```python
from build123d import *

# Parameters (mm, degrees)
F0_R            = 6.035
F1_DEPTH        = 3.175
F3_COPIES_COUNT = 2
F4_T3_ANGLE     = 67.6677552602
F4_T6_ANGLE     = 67.6677552602
F4_T9_ANGLE     = 135.3490310549
F4_T18_ANGLE    = 135.3490310549
F4_T21_ANGLE    = 67.6677552602
F4_T24_ANGLE    = 67.6677552602
F5_R            = 1.27


# Not quite as in the source:
# - a fillet or chamfer that OpenCascade refuses, or shapes differently, is made with other operations: its cross-section is extruded or revolved along the edge and cut away or added
# - a pattern or mirror of a feature is missing from the dataset's text; its kind, count and spacing are read off the source's solid


with BuildPart() as f1:
    # F0 (on Top) → F1 (new body, symmetric)
    with BuildSketch(Plane.XY):
        with BuildLine():
            Line((18.2389864028, 12.7), (-18.2389864028, 12.7))
            ThreePointArc((-18.2389864028, 12.7), (-22.225, 0), (-18.2389864028, -12.7))
            Line((-18.2389864028, -12.7), (18.2389864028, -12.7))
            ThreePointArc((18.2389864028, -12.7), (22.225, 0), (18.2389864028, 12.7))
        make_face()
        Circle(F0_R, mode=Mode.SUBTRACT)
    extrude(amount=F1_DEPTH, both=True)

    # F2 (on Front) → F3 (revolve, cut)
    with BuildSketch(Plane.XZ):
        with BuildLine():
            ThreePointArc((15.3565955658, 1.25), (17.1329395143, 3.0989826153), (17.78, 5.58))
            ThreePointArc((17.78, 5.58), (13.844578608, 10.5293777195), (8.1357717283, 7.8102960081))
            ThreePointArc((8.1357717283, 7.8102960081), (7.8220449826, 4.1615660577), (10.0434044342, 1.25))
            Line((10.0434044342, 1.25), (12.7, 1.25))
            Line((12.7, 1.25), (15.3565955658, 1.25))
        make_face()
        with BuildLine():
            ThreePointArc((10.0434044342, 1.25), (7.8220449826, 4.1615660577), (8.1357717283, 7.8102960081))
            Line((8.1357717283, 7.8102960081), (0, 7.8102960081))
            Line((0, 7.8102960081), (0, 1.25))
            Line((0, 1.25), (10.0434044342, 1.25))
        make_face()
        with BuildLine():
            ThreePointArc((12.7, 0.5), (14.0802173742, 0.6910941919), (15.3565955658, 1.25))
            Line((15.3565955658, 1.25), (12.7, 1.25))
            Line((12.7, 1.25), (12.7, 0.5))
        make_face()
        with BuildLine():
            Line((12.7, 1.25), (10.0434044342, 1.25))
            ThreePointArc((10.0434044342, 1.25), (11.3197826258, 0.6910941919), (12.7, 0.5))
            Line((12.7, 0.5), (12.7, 1.25))
        make_face()
    f3 = revolve(axis=Axis((0, 0, 0), (0, 0, -1)), mode=Mode.SUBTRACT)

    # F3_copies: F3 ×2 about axis
    f3_copies_axis = Axis((0, 0, 0), (1, 0, 0))
    for i in range(1, F3_COPIES_COUNT):
        add(f3.rotate(f3_copies_axis, i * 360 / F3_COPIES_COUNT), mode=Mode.SUBTRACT)

    # F4: fillet of radius 5.08 on 9 edges, made by hand


with BuildPart() as f4_tool1:
    # F4_s2 → F4_t3 (revolve)
    with BuildSketch(Plane(origin=(0, 0, 0), x_dir=(0, 0, 1), z_dir=(-0.9249960227, -0.379976786, 0))):
        with BuildLine():
            ThreePointArc((1.8375, -16.1351264533), (2.828830373, -17.7270898644), (3.175, -19.5702529066))
            Line((3.175, -19.5702529066), (3.175, -17.1746368568))
            ThreePointArc((3.175, -17.1746368568), (2.4626157548, -16.7110242417), (1.8375, -16.1351264533))
        make_face()
    revolve(axis=Axis((0, 0, 3.175), (0, 0, 1)), revolution_arc=F4_T3_ANGLE)


with BuildPart() as f4_tool4:
    # F4_s5 → F4_t6 (revolve)
    with BuildSketch(Plane.XZ):
        with BuildLine():
            ThreePointArc((16.1351264533, 1.8375), (17.7270898644, 2.828830373), (19.5702529066, 3.175))
            Line((19.5702529066, 3.175), (17.1746368568, 3.175))
            ThreePointArc((17.1746368568, 3.175), (16.7110242417, 2.4626157548), (16.1351264533, 1.8375))
        make_face()
    revolve(axis=Axis((0, 0, 3.175), (0, 0, 1)), revolution_arc=F4_T6_ANGLE)


with BuildPart() as f4_tool7:
    # F4_s8 → F4_t9 (revolve)
    with BuildSketch(Plane(origin=(0, 0, 0), x_dir=(0, 0, 1), z_dir=(0.9250408493, 0.3798676441, 0))):
        with BuildLine():
            ThreePointArc((1.8375, -16.1351264533), (2.828830373, -17.7270898644), (3.175, -19.5702529066))
            Line((3.175, -19.5702529066), (3.175, -17.1746368568))
            ThreePointArc((3.175, -17.1746368568), (2.4626157548, -16.7110242417), (1.8375, -16.1351264533))
        make_face()
    revolve(axis=Axis((0, 0, 3.175), (0, 0, 1)), revolution_arc=F4_T9_ANGLE)


with BuildPart() as f4_tool10:
    # F4_s11 → F4_t12 (revolve)
    with BuildSketch(Plane.XZ):
        with BuildLine():
            ThreePointArc((10.7844387246, 0.875), (9.8448385139, 1.1553685922), (8.8688774491, 1.25))
            Line((8.8688774491, 1.25), (10.0434044342, 1.25))
            ThreePointArc((10.0434044342, 1.25), (10.4062452626, 1.0473308962), (10.7844387246, 0.875))
        make_face()
    revolve(axis=Axis((0, 0, 1.25), (0, 0, -1)))


with BuildPart() as f4_tool13:
    # F4_s14 → F4_t15 (revolve)
    with BuildSketch(Plane.XZ):
        with BuildLine():
            ThreePointArc((8.8688774491, -1.25), (9.8448385139, -1.1553685922), (10.7844387245, -0.875))
            ThreePointArc((10.7844387245, -0.875), (10.4062452626, -1.0473308962), (10.0434044342, -1.25))
            Line((10.0434044342, -1.25), (8.8688774491, -1.25))
        make_face()
    revolve(axis=Axis((0, 0, -1.25), (0, 0, 1)))


with BuildPart() as f4_tool16:
    # F4_s17 → F4_t18 (revolve)
    with BuildSketch(Plane(origin=(0, 0, 0), x_dir=(0, 0, 1), z_dir=(0.9250408493, -0.3798676441, 0))):
        with BuildLine():
            ThreePointArc((-3.175, 19.5702529066), (-2.828830373, 17.7270898644), (-1.8375, 16.1351264533))
            ThreePointArc((-1.8375, 16.1351264533), (-2.4626157548, 16.7110242417), (-3.175, 17.1746368568))
            Line((-3.175, 17.1746368568), (-3.175, 19.5702529066))
        make_face()
    revolve(axis=Axis((0, 0, -3.175), (0, 0, -1)), revolution_arc=F4_T18_ANGLE)


with BuildPart() as f4_tool19:
    # F4_s20 → F4_t21 (revolve)
    with BuildSketch(Plane.XZ):
        with BuildLine():
            ThreePointArc((16.1351264533, -1.8375), (17.7270898644, -2.828830373), (19.5702529066, -3.175))
            Line((19.5702529066, -3.175), (17.1746368568, -3.175))
            ThreePointArc((17.1746368568, -3.175), (16.7110242417, -2.4626157548), (16.1351264533, -1.8375))
        make_face()
    revolve(axis=Axis((0, 0, -3.175), (0, 0, -1)), revolution_arc=F4_T21_ANGLE)


with BuildPart() as f4_tool22:
    # F4_s23 → F4_t24 (revolve)
    with BuildSketch(Plane(origin=(0, 0, 0), x_dir=(0, 0, 1), z_dir=(-0.9249960227, 0.379976786, 0))):
        with BuildLine():
            ThreePointArc((-1.8375, 16.1351264533), (-2.828830373, 17.7270898644), (-3.175, 19.5702529066))
            Line((-3.175, 19.5702529066), (-3.175, 17.1746368568))
            ThreePointArc((-3.175, 17.1746368568), (-2.4626157548, 16.7110242417), (-1.8375, 16.1351264533))
        make_face()
    revolve(axis=Axis((0, 0, -3.175), (0, 0, -1)), revolution_arc=F4_T24_ANGLE)


with BuildPart() as f1_1:
    add(f1.part)

    # F4_t25: cut F4_tool1, F4_tool4, F4_tool7, F4_tool10, F4_tool13, F4_tool16, F4_tool19, F4_tool22
    add([f4_tool1.part, f4_tool4.part, f4_tool7.part, f4_tool10.part, f4_tool13.part, f4_tool16.part, f4_tool19.part, f4_tool22.part], mode=Mode.SUBTRACT)

    # F5
    f5_edges = [f1_1.edges().sort_by_distance(p)[0] for p in [
        (-18.238986, -12.7, 0),
        (-18.238986, 12.7, 0),
        (18.238986, 12.7, 0),
        (18.238986, -12.7, 0),
    ]]
    fillet(f5_edges, radius=F5_R)


solid = f1_1.part
```
Geometry: final body of the model. Coordinates: model frame, mm. Round coordinates to 2 decimals unless told otherwise and drop trailing zeros. Order: outer loops, then holes, each group sorted by start corner. A loop starts at its lowest first (then second) coordinate and runs counter-clockwise, first axis right, second up. Notation, with made-up numbers: M -8,-33.5 L -4,-33.5 A28 cw -4,5.5 Z; hole C 47.25,19.25 d7. An arc over 180 degrees is marked long. Use one line per item in the form item = value. Start each with the question number.
Q1. Cut plane A-A (z = -2.5). Return loops of the section in (x, y) (3 decimals), and give its area (3 significant figures).
Q2. Material intervals for line 1 (X direction, y = 0, z = -0.1) (3 decimals); line 2 (Y direction, x = 0, z = 0) (3 decimals); line 3 (Z direction, x = 5, y = -6.5), sorted ascending. Write a range as [from, to].
Q3. Mould query, pull axis X, two halves, no side actions, for faces 1 (the face through (-18.16, 12.55, 0.04)), 2 (the face through (-6, -2, -1.25)), 3 (the face through (18.16, 12.55, -0.04)). Classes: +X half, -X half, draft (parallel to the pull), parting line (faces both ways), or undercut.
Q4. Pin query (flat end, axial travel): pin 1 Ø12 at (x, y) = (6, 2.5) entering from +Z; pin 2 Ø1 at (x, y) = (10, 6.5) entering from +Z; pin 3 Ø3 at (y, z) = (4, 2) entering from -X. Return the tip coordinate at first contact, or that it passes through.
Geometry results:
q1.outline = M -18.628,-12.123 A1.27 ccw -17.563,-12.7 L -11.361,-12.7 A17.04 cw -11.361,12.7 L -17.563,12.7 A1.27 ccw -18.628,12.123 A22.225 ccw Z; M 11.361,-12.7 L 17.563,-12.7 A1.27 ccw 18.628,-12.123 A22.225 ccw 18.628,12.123 A1.27 ccw 17.563,12.7 L 11.361,12.7 A17.04 cw Z
q1.area = 287 mm^2
q2.line_1 = [-22.225, -6.035], [6.035, 22.225]
q2.line_2 = [-12.7, -6.035], [6.035, 12.7]
q2.line_3 = [-1.25, 1.25]
q3.face_1 = -X half
q3.face_2 = undercut
q3.face_3 = +X half
q4.pin_1 = 1.25
q4.pin_2 = 0.66
q4.pin_3 = -22.08
